Source: CAD feature listing. Evaluate the final solid. Frame: model axes, mm. A direction names the side the tool comes from. Coordinates: 2 decimals unless noted, no trailing zeros. Order: outer loops, then holes, each group sorted by start corner. A loop starts at its lowest first (then second) coordinate and runs counter-clockwise, first axis right, second up. Notation, with made-up numbers: (63, -5.75) - (85, -5.75) arc R20 ccw to (85, 20.25) - close; hole circle Ø8 at (59, -28.75). An arc over 180 degrees is marked (long way). One line per question, with ' | ' between items.
from build123d import *

# Parameters (mm, degrees)
F1_DEPTH     = 63.5
F2_T         = -5.08
F3_R         = 5.08
F4_DEPTH     = 38.1
F5_T1_DEPTH  = 311.15
F5_T3_DEPTH  = 266.7
F5_T5_DEPTH  = 152.4
F5_T8_ANGLE  = 90
F5_T10_ANGLE = 90


# Not quite as in the source:
# - a fillet or chamfer that OpenCascade refuses, or shapes differently, is made with other operations: its cross-section is extruded or revolved along the edge and cut away or added


with BuildPart() as f1:
    # F0 (on Top) → F1 (new body)
    with BuildSketch(Plane.XY):
        with BuildLine():
            Line((-344.2945734978, 176.2892417401), (-401.1594021572, 176.2892417401))
            Line((-401.1594021572, 176.2892417401), (-401.1594021572, -26.9107582599))
            Line((-401.1594021572, -26.9107582599), (-344.2945734978, -26.9107582599))
            Line((-344.2945734978, -26.9107582599), (-121.7594021572, -26.9107582599))
            ThreePointArc((-121.7594021572, -26.9107582599), (-103.7988899151, -19.471270502), (-96.3594021572, -1.5107582599))
            Line((-96.3594021572, -1.5107582599), (-96.3594021572, 6.5090437472))
            Line((-96.3594021572, 6.5090437472), (-96.3594021572, 44.6090437472))
            Line((-96.3594021572, 44.6090437472), (-96.3594021572, 150.8892417401))
            ThreePointArc((-96.3594021572, 150.8892417401), (-103.7988899151, 168.8497539822), (-121.7594021572, 176.2892417401))
            Line((-121.7594021572, 176.2892417401), (-344.2945734978, 176.2892417401))
        make_face()
    extrude(amount=F1_DEPTH)

    # F2
    f2_openings = [f1.faces().sort_by_distance(p)[0] for p in [
        (-249.418343, 74.689242, 63.5),
        (-401.159402, 74.689242, 31.75),
    ]]
    offset(amount=F2_T, openings=f2_openings)

    # F3 (on face) → F4 (join)
    with BuildSketch(Plane.YZ.offset(-96.3594021572)):
        with Locations((74.6892417401, 38.1)):
            Circle(F3_R)
    extrude(amount=F4_DEPTH)

    # F5: fillet of radius 12.7 on 6 edges, made by hand

    # F5_s2 → F5_t1 (cut)
    with BuildSketch(Plane.YZ.offset(-432.9094021572)):
        with BuildLine():
            ThreePointArc((176.2892417401, 12.7), (172.5694978612, 3.7197438789), (163.5892417401, 0))
            Line((163.5892417401, 0), (176.2892417401, 0))
            Line((176.2892417401, 0), (176.2892417401, 12.7))
        make_face()
        with BuildLine():
            ThreePointArc((-14.2107582599, 0), (-23.191014381, 3.7197438789), (-26.9107582599, 12.7))
            Line((-26.9107582599, 12.7), (-26.9107582599, 0))
            Line((-26.9107582599, 0), (-14.2107582599, 0))
        make_face()
    extrude(amount=F5_T1_DEPTH, mode=Mode.SUBTRACT)

    # F5_s4 → F5_t3 (cut)
    with BuildSketch(Plane.XZ.offset(-208.0392417401)):
        with BuildLine():
            ThreePointArc((-401.1594021572, 12.7), (-397.4396582783, 3.7197438789), (-388.4594021572, 0))
            Line((-388.4594021572, 0), (-401.1594021572, 0))
            Line((-401.1594021572, 0), (-401.1594021572, 12.7))
        make_face()
    extrude(amount=F5_T3_DEPTH, mode=Mode.SUBTRACT)

    # F5_s6 → F5_t5 (cut)
    with BuildSketch(Plane.XZ.offset(-150.8892417401)):
        with BuildLine():
            ThreePointArc((-109.0594021572, 0), (-100.0791460361, 3.7197438789), (-96.3594021572, 12.7))
            Line((-96.3594021572, 12.7), (-96.3594021572, 0))
            Line((-96.3594021572, 0), (-109.0594021572, 0))
        make_face()
    extrude(amount=F5_T5_DEPTH, mode=Mode.SUBTRACT)

    # F5_s7 → F5_t8 (revolve, cut)
    with BuildSketch(Plane.YZ.offset(-121.7594021572)):
        with BuildLine():
            ThreePointArc((-14.2107582599, 0), (-23.191014381, 3.7197438789), (-26.9107582599, 12.7))
            Line((-26.9107582599, 12.7), (-26.9107582599, 0))
            Line((-26.9107582599, 0), (-14.2107582599, 0))
        make_face()
    revolve(axis=Axis((-121.7594021572, -1.5107582599, 0), (0, 0, 1)), revolution_arc=F5_T8_ANGLE, mode=Mode.SUBTRACT)

    # F5_s9 → F5_t10 (revolve, cut)
    with BuildSketch(Plane.XZ.offset(-150.8892417401)):
        with BuildLine():
            ThreePointArc((-96.3594021572, 12.7), (-100.0791460361, 3.7197438789), (-109.0594021572, 0))
            Line((-109.0594021572, 0), (-96.3594021572, 0))
            Line((-96.3594021572, 0), (-96.3594021572, 12.7))
        make_face()
    revolve(axis=Axis((-121.7594021572, 150.8892417401, 0), (0, 0, 1)), revolution_arc=F5_T10_ANGLE, mode=Mode.SUBTRACT)


solid = f1.part
(1) Cut plane D-D (x = -87). Return the cut outline in (y, z).
Taken from the geometry:
outline: circle Ø10.16 at (74.69, 38.1)
(2) Cut plane B-B (x = -307). Return the cut outline in (y, z).
Taken from the geometry:
outline: (-26.91, 12.7) arc R12.7 ccw to (-14.21, 0) - (163.59, 0) arc R12.7 ccw to (176.29, 12.7) - (176.29, 63.5) - (171.21, 63.5) - (171.21, 5.08) - (-21.83, 5.08) - (-21.83, 63.5) - (-26.91, 63.5) - close
(3) Cut plane C-C (y = 5.5). Return the cut outline in (x, z), and give its area (3 significant figures).
Taken from the geometry:
outline: (-398.62, 5.08) arc R12.7 ccw to (-388.46, 0) - (-109.06, 0) arc R12.7 ccw to (-96.36, 12.7) - (-96.36, 63.5) - (-101.44, 63.5) - (-101.44, 5.08) - close | area: 1,780 mm²
(4) Cut plane A-A (z = 38.1). Return the cut outline in (x, y).
Taken from the geometry:
outline: (-401.16, -26.91) - (-121.76, -26.91) arc R25.4 ccw to (-96.36, -1.51) - (-96.36, 69.61) - (-58.26, 69.61) - (-58.26, 79.77) - (-96.36, 79.77) - (-96.36, 150.89) arc R25.4 ccw to (-121.76, 176.29) - (-401.16, 176.29) - (-401.16, 171.21) - (-121.76, 171.21) arc R20.32 cw to (-101.44, 150.89) - (-101.44, -1.51) arc R20.32 cw to (-121.76, -21.83) - (-401.16, -21.83) - close
(5) Material intervals for L1, parallel to Y at x = -236.5, z = 34.5; L2, parallel to Z at x = -197, y = 77; L3, parallel to X at y = 72.5, z = 53.5, sorted ascending. Write a range as from..to.
Taken from the geometry:
L1: y = -26.91..-21.83, 171.21..176.29 | L2: z = 0..5.08 | L3: x = -101.44..-96.36
(6) Pin query (flat end, axial travel): P1, Ø12, axis at y = 87.5, z = 16, coming from the -X side; P2, Ø1, axis at x = -284.5, y = 15.5, coming from the +Z side; P3, Ø8, axis at y = 71.5, z = 15, coming from the +X side. Return the tip coordinate at first contact, or that it passes through.
Taken from the geometry:
P1: stops at x = -101.44 | P2: stops at z = 5.08 | P3: stops at x = -96.36
(7) Set-up query: faces 1 (the cylindrical face through (-107.55, -16.036, 33.881)), 2 (the cylindrical face through (-77.576, 70.658, 35.009)), 3 (the cylindrical face through (-393.95, 76.11, 1.25)). Return all of +Z, -Z, +X, -X, +Y, -Y with unobstructed straight access to the full face (end or side cutting, diameter ignored); none if empty.
Taken from the geometry:
face 1: +Z, -X | face 2: +X | face 3: -Z, -X, +Y, -Y
(8) Pull-direction query (Y, two-part tool) for faces 4 (the cylindrical face through (-104, -19.67, 37.74)), 5 (the cylindrical face through (-107.234, 165.099, 33.881)), 6 (the cylindrical face through (-263.42, 172.67, 3.82)), 7 (the flat face through (-58.259, 75, 38)); classes: pulls with the +Y half, pulls with the -Y half, needs draft (parallel to the pull), parting line crosses it, or undercut.
Taken from the geometry:
face 4: pulls with the -Y half | face 5: undercut | face 6: pulls with the +Y half | face 7: needs draft
